```python
from build123d import *

# Parameters (mm, degrees)
PAD_DEPTH           = 10
HOLE001_D           = 5
HOLE001_DEPTH       = 195.23
HOLE001_CSINK_D     = 9
HOLE001_CSINK_ANGLE = 90


with BuildPart() as part:
    # Sketch → Pad (new body)
    with BuildSketch(Plane.XZ):
        with BuildLine():
            Line((-37.345, 0), (-37.345, -38.855))
            Line((-37.345, -38.855), (-25.641107, -27.151107))
            ThreePointArc((-25.641107, -27.151107), (26.781742, -26.026665), (26.406903, 26.406903))
            ThreePointArc((26.406903, 26.406903), (21.103602, 26.406903), (21.103602, 21.103602))
            ThreePointArc((-29.845, 0), (11.421187, -27.573185), (21.103602, 21.103602))
            ThreePointArc((-29.845, 0), (-33.595, 3.75), (-37.345, 0))
        make_face()
    extrude(amount=PAD_DEPTH)

    # Hole001
    with Locations(Plane(origin=(0.755, 0, -0.755), x_dir=(0.707107, 0, 0.707107), z_dir=(0.707107, 0, -0.707107))):
        with Locations((-45.605635, 5)):
            CounterSinkHole(HOLE001_D / 2, HOLE001_CSINK_D / 2, depth=HOLE001_DEPTH, counter_sink_angle=HOLE001_CSINK_ANGLE)


solid = part.part
```
Input: part model. Units: mm. Frame: model coordinates. Coordinates: 2 decimals unless noted, no trailing zeros. Loops run counter-clockwise (first coordinate to the right, second up) from the corner with the lowest first, then second, coordinate; pieces in that order, holes last.
Q1. Section C-C, the plane z = -17. Return the cut outline in (x, y) (3 decimals), and give its area (3 significant figures).
Results are:
outline: (-37.345, -10) - (-24.53, -10) - (-24.53, 0) - (-37.345, 0) - close; (24.53, -10) - (33.251, -10) - (33.251, 0) - (24.53, 0) - close
area: 215 mm2
Q2. Section A-A, the plane z = -3. Return the cut outline in (x, y) (3 decimals).
Results are:
outline: (-37.345, -10) - (-29.694, -10) - (-29.694, 0) - (-37.345, 0) - close; (29.694, -10) - (37.224, -10) - (37.224, 0) - (29.694, 0) - close
Q3. Section B-B, the plane x = 0. Return the cut outline in (y, z) (3 decimals).
Results are:
outline: (-10, -37.345) - (0, -37.345) - (0, -29.845) - (-10, -29.845) - close
Q4. Contact query for flat-ended pins moving along their axis: pin 1 (1.5 mm diameter, centred on x = 5.5, y = -7, fed in from +Z); pin 2 (6 mm diameter, centred on y = -8, z = -28, fed in from +X); pin 3 (5 mm diameter, centred on x = 25, z = 11, fed in from +Y); pin 4 (5 mm diameter, centred on y = -4, z = 19, fed in from +X). Output: stop coordinate, or through.
Results are:
pin 1: stops at z = -29.18
pin 2: stops at x = 27.74
pin 3: passes through
pin 4: stops at x = 33.5
Q5. Mould query, pull axis Y, two halves, no side actions, for faces 1 (the flat face through (-32.88, -0.49, -34.39)), 2 (the cylindrical face through (-33.627, -5.11, -27.337)), 3 (the flat face through (3, -10, -30)). Classes: +Y half, -Y half, draft (parallel to the pull), parting line (faces both ways), or undercut.
Results are:
face 1: draft
face 2: undercut
face 3: -Y half
Q6. Line query: line 1 along Z through (x, y) = (0, -4.5) (3 decimals); line 2 along Z through (x, y) = (24.5, -4.5); line 3 along X through (y, z) = (-8.75, -9) (3 decimals). Output: solid intervals per line, ascending.
Results are:
line 1: z = -37.345 to -29.845
line 2: z = -28.19 to -17.04, 17.04 to 27.43
line 3: x = -37.345 to -28.456, 28.456 to 36.244
Q7. Section D-D, the plane z = 17. Return the cut outline in (x, y).
Results are:
outline: (24.53, -10) - (33.25, -10) - (33.25, 0) - (24.53, 0) - close
